Autodesk Inventor part; units mm, degrees
ref_plane "YZ Plane" through (0, 0, 0) normal (1, 0, 0) x (0, 1, 0)
ref_plane "XZ Plane" through (0, 0, 0) normal (0, 1, 0) x (-1, 0, 0)
ref_plane "XY Plane" through (0, 0, 0) normal (0, 0, 1) x (1, 0, 0)
sketch "Sketch1" plane through (0, 0, 0) normal (0, 1, 0) x (-1, 0, 0)
  circle A0 centre (0, 0) radius 26.6
  line L0 (0, -26.6) -> (0, -74.6) construction
  line L1 (-44.5, -74.6) -> (44.5, -74.6)
  line L2 (0, 26.6) -> (0, 68.1) construction
  line L3 (-44.5, -74.6) -> (-63.8947, -24.9684)
  line L4 (26.6, 0) -> (69.1, 0) construction
  arc A1 (-8.2674, 68.1) -> (-63.8947, -24.9684) centre (0, 0) ccw
  line L5 (44.5, -74.6) -> (44.5, -70.6)
  line L6 (56.5, -58.6) -> (60.923, -58.6)
  arc A2 (56.5, -58.6) -> (44.5, -70.6) centre (56.5, -70.6) ccw
  arc A3 (60.923, -58.6) -> (68.923, -50.6) centre (60.923, -50.6) ccw
  line L7 (68.923, 68.1) -> (27.423, 68.1) construction
  line L8 (27.423, 68.1) -> (27.423, 62.6) construction
  line L9 (31.423, 62.6) -> (68.923, 62.6)
  line L10 (-8.2674, 68.1) -> (23.923, 68.1)
  line L11 (27.423, 66.6) -> (27.423, 64.6)
  line L12 (68.923, 62.6) -> (68.923, -50.6)
  arc A4 (27.423, 64.6) -> (23.923, 68.1) centre (23.923, 64.6) ccw
  arc A5 (27.423, 66.6) -> (31.423, 62.6) centre (31.423, 66.6) ccw
  point P0 (44.5, -58.6)
  dimension "d0" = 53.2
  dimension "d2" = 48
  dimension "d3" = 44.5
  dimension "d4" = 89
  dimension "d5" = 41.5
  dimension "d6" = 42.5
  dimension "d7" = 16
  dimension "d8" = 12
  dimension "d9" = 8
  dimension "d10" = 5.5
  dimension "d11" = 41.5
  dimension "d12" = 3.5
  dimension "d13" = 4
extrude "Extrusion1" add sketch "Sketch1" along normal blind 50.5
sketch "Sketch2" plane through (0, 50.5, 0) normal (0, 1, 0) x (1, 0, 0)
  circle A0 centre (0, 0) radius 45
  dimension "d16" = 90
extrude "Extrusion2" cut sketch "Sketch2" against normal blind 26
sketch "Sketch3" plane through (0, 0, 0) normal (0, 0, 1) x (1, 0, 0)
  line L0 (68.6, 22.5) -> (85.1798, 22.5)
  line L1 (68.6, 0) -> (50.1, 0)
  line L2 (68.6, 0) -> (8.2674, 0)
  line L3 (50.1, 0) -> (68.6, 22.5)
  line L4 (68.6, 0) -> (85.1798, 22.5)
  point P0 (0, 0)
  point P1 (63.8947, 0)
  dimension "d20" = 18.5
extrude "Extrusion3" cut sketch "Sketch3" along normal mid plane 150
properties part number "PocketNC_Workpiece_Z_axis_rotation"
For this review, take the finished solid that the model builds, in its own axes (mm). A direction names the side the tool comes from. Coordinates: 2 decimals unless noted, no trailing zeros. Loops run counter-clockwise (first coordinate to the right, second up) from the corner with the lowest first, then second, coordinate; pieces in that order, holes last. Notation, with made-up numbers: (-30, -11) -> (-16, -11) arc R7 ccw to (-16, -3) -> close; hole circle Ø1 at (25, 12). An arc over 180 degrees is marked (long way). Write each question's results on one line, items separated by ' | '.
Q1. Add section C-C, the plane y = 47. State the section outline as (x, z) points, then the cut area to 3 significant figures.
Taken from the geometry:
outline: (-68.92, -50.6) arc R8 ccw to (-60.92, -58.6) -> (-56.5, -58.6) arc R12 cw to (-44.5, -70.6) -> (-44.5, -74.6) -> (44.5, -74.6) -> (63.89, -24.97) arc R68.6 ccw to (8.27, 68.1) -> (-23.92, 68.1) arc R3.5 ccw to (-27.42, 64.6) -> (-27.42, 66.6) arc R4 cw to (-31.42, 62.6) -> (-68.92, 62.6) -> close; hole circle Ø90 at (0, 0) | area: 10,900 mm²
Q2. Mouldability with a two-part tool opening along X and no side actions: class faces 4 (the flat face through (57.165, 8.592, -7.454)), 5 (the cylindrical face through (-12.27, 12.08, 23.6)), 6 (the flat face through (-22, 0, -18)) as +X half, -X half, draft (parallel to the pull), parting line (faces both ways), or undercut.
Taken from the geometry:
face 4: +X half | face 5: undercut | face 6: draft
Q3. To check wall thickness, follow line 1 along Z through (x, y) = (0, 12); line 2 along Z through (x, y) = (0, 41); line 3 along X through (y, z) = (38, 0). State the ranges of each line that lie inside material, in increasing order. Write a range as [from, to].
Taken from the geometry:
line 1: [-74.6, -26.6], [26.6, 68.1] | line 2: [-74.6, -45], [45, 68.1] | line 3: [-68.92, -45], [45, 68.6]
Q4. Machinability: for faces 1 (the flat face through (19, 24.5, 19)), 2 (the flat face through (-59, 25, -58.6)), 3 (the flat face through (-50, 25, 62.6)), which of the approach directions +Z, -Z, +X, -X, +Y, -Y give a long, thin tool a straight path to every point of the face, cutting with its end or side? Answer none if there is none.
Taken from the geometry:
face 1: +Y | face 2: -Z, -X, +Y, -Y | face 3: +Z, -X, +Y, -Y
Q5. Add section D-D, the plane x = -37.5. State the section outline as (y, z) points.
Taken from the geometry:
outline: (0, -74.6) -> (50.5, -74.6) -> (50.5, -24.87) -> (24.5, -24.87) -> (24.5, 24.87) -> (50.5, 24.87) -> (50.5, 62.6) -> (0, 62.6) -> close
Q6. Add section B-B, the plane z = 0. State the section outline as (x, y) points.
Taken from the geometry:
outline: (-68.92, 0) -> (-26.6, 0) -> (-26.6, 24.5) -> (-45, 24.5) -> (-45, 50.5) -> (-68.92, 50.5) -> close; (26.6, 0) -> (50.1, 0) -> (68.6, 22.5) -> (68.6, 50.5) -> (45, 50.5) -> (45, 24.5) -> (26.6, 24.5) -> close
Q7. For pin 1 Ø6 at (x, y) = (-53, 25.5) entering from -Z; pin 2 Ø2 at (x, z) = (-41, -3) entering from +Y; pin 3 Ø2 at (y, z) = (32, -56.5) entering from +X; pin 4 Ø3 at (x, z) = (-43, 26.5) entering from -Y, all flat-tipped, find the tip position at first contact; note any pin that passes through.
Taken from the geometry:
pin 1: z = -60.51 | pin 2: y = 24.5 | pin 3: x = 51.96 | pin 4: y = 0
Q8. Add section A-A, the plane x = 0. State the section outline as (y, z) points.
Taken from the geometry:
outline: (0, -74.6) -> (50.5, -74.6) -> (50.5, -45) -> (24.5, -45) -> (24.5, -26.6) -> (0, -26.6) -> close; (0, 26.6) -> (24.5, 26.6) -> (24.5, 45) -> (50.5, 45) -> (50.5, 68.1) -> (0, 68.1) -> close
